Geometry: final body of the model. Coordinates: model frame, mm. Face numbers are marked on the shaded views. Round coordinates to 2 decimals unless told otherwise and drop trailing zeros. Loops run counter-clockwise (first coordinate to the right, second up) from the corner with the lowest first, then second, coordinate; pieces in that order, holes last. Notation, with made-up numbers: (75, 18) - (123, 18) arc R20 cw to (123, 38) - close; hole circle Ø8 at (28.5, 74.25). An arc over 180 degrees is marked (long way). Answer in a Markdown table with one row per item. Add a question column.
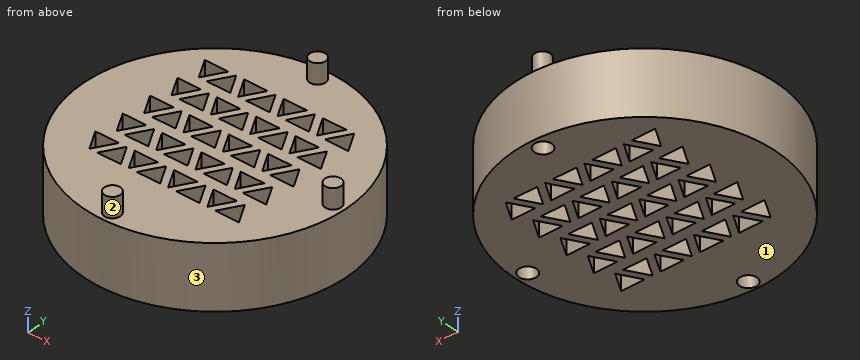
from build123d import *

# Parameters (mm, degrees)
F0_R     = 16.5
F1_DEPTH = 8
F2_R     = 1.1
F3_DEPTH = 2.5
F4_R     = 1
F5_DEPTH = 2.5
F7_DEPTH = 25


with BuildPart() as f1:
    # F0 (on Top) → F1 (new body)
    with BuildSketch(Plane.XY):
        Circle(F0_R)
    extrude(amount=F1_DEPTH)

    # F2 (on face) → F3 (cut)
    with BuildSketch(Plane(origin=(0, 0, 0), x_dir=(1, 0, 0), z_dir=(0, 0, -1))):
        with Locations((0, 15.1)):
            Circle(F2_R)
        with Locations((15, 0.1)):
            Circle(F2_R)
        with Locations((0, -14.9)):
            Circle(F2_R)
    extrude(amount=-F3_DEPTH, mode=Mode.SUBTRACT)

    # F4 (on face) → F5 (join)
    with BuildSketch(Plane.XY.offset(8)):
        with Locations((0, 15)):
            Circle(F4_R)
        with Locations((15, 0)):
            Circle(F4_R)
        with Locations((0, -15)):
            Circle(F4_R)
    extrude(amount=F5_DEPTH)

    # F6 (on face) → F7 (cut)
    with BuildSketch(Plane.XY.offset(8)):
        Polygon((-7.25, -5.700962), (-10.25, -5.700962), (-8.75, -8.299038), align=None)
        Polygon((-6.25, -5.700962), (-7.75, -8.299038), (-4.75, -8.299038), align=None)
        Polygon((-7.25, -1.700962), (-10.25, -1.700962), (-8.75, -4.299038), align=None)
        Polygon((-6.25, -1.700962), (-7.75, -4.299038), (-4.75, -4.299038), align=None)
        Polygon((-7.25, 2.299038), (-10.25, 2.299038), (-8.75, -0.299038), align=None)
        Polygon((-6.25, 2.299038), (-7.75, -0.299038), (-4.75, -0.299038), align=None)
        Polygon((-7.25, 6.299038), (-10.25, 6.299038), (-8.75, 3.700962), align=None)
        Polygon((-6.25, 6.299038), (-7.75, 3.700962), (-4.75, 3.700962), align=None)
        Polygon((-7.25, 10.299038), (-10.25, 10.299038), (-8.75, 7.700962), align=None)
        Polygon((-6.25, 10.299038), (-7.75, 7.700962), (-4.75, 7.700962), align=None)
        Polygon((-2.25, -5.700962), (-5.25, -5.700962), (-3.75, -8.299038), align=None)
        Polygon((-1.25, -5.700962), (-2.75, -8.299038), (0.25, -8.299038), align=None)
        Polygon((-2.25, -1.700962), (-5.25, -1.700962), (-3.75, -4.299038), align=None)
        Polygon((-1.25, -1.700962), (-2.75, -4.299038), (0.25, -4.299038), align=None)
        Polygon((-2.25, 2.299038), (-5.25, 2.299038), (-3.75, -0.299038), align=None)
        Polygon((-1.25, 2.299038), (-2.75, -0.299038), (0.25, -0.299038), align=None)
        Polygon((-2.25, 6.299038), (-5.25, 6.299038), (-3.75, 3.700962), align=None)
        Polygon((-1.25, 6.299038), (-2.75, 3.700962), (0.25, 3.700962), align=None)
        Polygon((-2.25, 10.299038), (-5.25, 10.299038), (-3.75, 7.700962), align=None)
        Polygon((-1.25, 10.299038), (-2.75, 7.700962), (0.25, 7.700962), align=None)
        Polygon((2.75, -5.700962), (-0.25, -5.700962), (1.25, -8.299038), align=None)
        Polygon((3.75, -5.700962), (2.25, -8.299038), (5.25, -8.299038), align=None)
        Polygon((2.75, -1.700962), (-0.25, -1.700962), (1.25, -4.299038), align=None)
        Polygon((3.75, -1.700962), (2.25, -4.299038), (5.25, -4.299038), align=None)
        Polygon((2.75, 2.299038), (-0.25, 2.299038), (1.25, -0.299038), align=None)
        Polygon((3.75, 2.299038), (2.25, -0.299038), (5.25, -0.299038), align=None)
        Polygon((2.75, 6.299038), (-0.25, 6.299038), (1.25, 3.700962), align=None)
        Polygon((3.75, 6.299038), (2.25, 3.700962), (5.25, 3.700962), align=None)
        Polygon((2.75, 10.299038), (-0.25, 10.299038), (1.25, 7.700962), align=None)
        Polygon((3.75, 10.299038), (2.25, 7.700962), (5.25, 7.700962), align=None)
        Polygon((7.75, -5.700962), (4.75, -5.700962), (6.25, -8.299038), align=None)
        Polygon((8.75, -5.700962), (7.25, -8.299038), (10.25, -8.299038), align=None)
        Polygon((7.75, -1.700962), (4.75, -1.700962), (6.25, -4.299038), align=None)
        Polygon((8.75, -1.700962), (7.25, -4.299038), (10.25, -4.299038), align=None)
        Polygon((7.75, 2.299038), (4.75, 2.299038), (6.25, -0.299038), align=None)
        Polygon((8.75, 2.299038), (7.25, -0.299038), (10.25, -0.299038), align=None)
        Polygon((7.75, 6.299038), (4.75, 6.299038), (6.25, 3.700962), align=None)
        Polygon((8.75, 6.299038), (7.25, 3.700962), (10.25, 3.700962), align=None)
        Polygon((7.75, 10.299038), (4.75, 10.299038), (6.25, 7.700962), align=None)
        Polygon((8.75, 10.299038), (7.25, 7.700962), (10.25, 7.700962), align=None)
    extrude(amount=-F7_DEPTH, mode=Mode.SUBTRACT)


solid = f1.part
1) Section C-C, the plane x = -14.5. Return the cut outline in (y, z), and give its area (3 significant figures).
2) Pull-direction query (Y, two-part tool) for the marked faces 1, 2 and 3; classes: pulls with the +Y half, pulls with the -Y half, needs draft (parallel to the pull), parting line crosses it, or undercut.
3) Section A-A, the plane z = 9.75. Return the cut outline in (x, y).
4) Section B-B, the plane z = 3. Give the number of separate pieces and of enclosed holes in the cut face, and give its area (3 significant figures).
5) Contact query for flat-ended pins moving along their axis: pin 1 Ø3.5 at (x, z) = (-4, 3) entering from -Y; pin 2 Ø2.5 at (x, z) = (6.5, 5) entering from -Y; pin 3 Ø1 at (x, z) = (-8, 9) entering from +Y; pin 4 Ø1 at (y, z) = (2.5, 3) entering from +X. Output: stop coordinate, or through.
6) Material intervals for line 1 along Y through (x, z) = (-3, 7.25); line 2 along Z through (x, y) = (0.5, 13); line 3 along X through (y, z) = (-15.1, 1), sorted ascending. Write a range as from..to.
Evaluation:
| question | item | result |
|---|---|---|
| 1 | outline | (-7.87, 0) - (7.87, 0) - (7.87, 8) - (-7.87, 8) - close |
| 1 | area | 126 mm² |
| 2 | face 1 | needs draft |
| 2 | face 2 | undercut |
| 2 | face 3 | parting line crosses it |
| 3 | outline | circle Ø2 at (0, -15); circle Ø2 at (0, 15); circle Ø2 at (15, 0) |
| 4 | separate pieces | 1 |
| 4 | enclosed holes | 40 |
| 4 | area | 699 mm² |
| 5 | pin 1 | stops at y = -16.35 |
| 5 | pin 2 | stops at y = -15.64 |
| 5 | pin 3 | passes through |
| 5 | pin 4 | stops at x = 16.38 |
| 6 | line 1 | y = -16.22..-7, -5.7..-3, -1.7..1, 2.3..5, 6.3..9, 10.3..16.22 |
| 6 | line 2 | z = 0..8 |
| 6 | line 3 | x = -6.65..-1.1, 1.1..6.65 |
